```python
from build123d import *

# Parameters (mm, degrees)
BOSS_EXTRUDE1_START = -70.140187
SKETCH1_R           = 68.58
SKETCH1_R_2         = 66.04
BOSS_EXTRUDE1_DEPTH = 70.140187
SKETCH2_R           = 3.175
SKETCH2_R_2         = 63.5
BOSS_EXTRUDE2_DEPTH = 1.5875


with BuildPart() as part:
    # Sketch1 → Boss-Extrude1 (new body)
    with BuildSketch(Plane.XY.offset(BOSS_EXTRUDE1_START)):
        with Locations((24.840813797, -46.264409372)):
            Circle(SKETCH1_R)
        with Locations((24.840813797, -46.264409372)):
            Circle(SKETCH1_R_2, mode=Mode.SUBTRACT)
    extrude(amount=BOSS_EXTRUDE1_DEPTH)

    # Sketch2 → Boss-Extrude2 (add)
    with BuildSketch(Plane(origin=(0, 0, -70.14018706), x_dir=(-1, 0, 0), z_dir=(0, 0, -1))):
        Polygon((0, -107.763073453), (107.763073453, 0), (0, 107.763073453), (-107.763073453, 0), align=None)
        with Locations((0, 98.782817332)):
            Circle(SKETCH2_R, mode=Mode.SUBTRACT)
        with Locations((98.782817332, 0)):
            Circle(SKETCH2_R, mode=Mode.SUBTRACT)
        with Locations((0, -98.782817332)):
            Circle(SKETCH2_R, mode=Mode.SUBTRACT)
        with Locations((-98.782817332, 0)):
            Circle(SKETCH2_R, mode=Mode.SUBTRACT)
        with Locations(Location((0, 0, 0), (0, 0, 173.121854306))):
            Circle(SKETCH2_R_2, mode=Mode.SUBTRACT)
    extrude(amount=BOSS_EXTRUDE2_DEPTH)


solid = part.part
```
Here's how the part is built. I have some questions about the finished solid (model axes, mm). A direction names the side the tool comes from. Give positions to 0.01 mm unless a question says otherwise; leave off trailing zeros. Loops run counter-clockwise (first coordinate to the right, second up) from the corner with the lowest first, then second, coordinate; pieces in that order, holes last. Notation, with made-up numbers: M 32,32.5 L 90,32.5 A8 ccw 90,38.5 Z; hole C 70.5,20.5 d11. An arc over 180 degrees is marked long. Use one line per item in the form item = value. Start each with the question number.
Q1. I need wall thicknesses on line 1 along Y through (x, z) = (0, -71.25); line 2 along Z through (x, y) = (71.5, -27); line 3 along X through (y, z) = (-76.5, -19.5). Which ranges of each line are inside material? Lowest first, please.
Q2. Which directions (+Z, -Z, +X, -X, +Y, -Y) give clear straight access to the entire face, cutting with the end or side of a thin tool? Please do faces 1 (the flat face through (23, -62, -70.14)), 2 (the flat face through (46, -109, -70.14)), 3 (the flat face through (-10, 11, -70.14)).
Q3. If we section it at B-B (y = -37): Write out the boundary of the cut face in (x, z).
Q4. If we section it at C-C (x = 11): Write out the boundary of the cut face in (y, z).
Q5. Will these pins go through, and if not, where does the flat tip stop? pin 1 Ø5 at (x, z) = (3.5, -17) entering from -Y; pin 2 Ø7.5 at (x, y) = (0, -98.78) entering from +Z; pin 3 Ø1.5 at (x, z) = (-10, -48) entering from -Y.
Q6. If we section it at A-A (x = 81.5): Write out the boundary of the cut face in (y, z), then the cut area to 3 significant figures.
Q7. If we section it at D-D (z = -12.5): Write out the boundary of the cut face in (x, y), then the cut area to 3 significant figures.
Q8. Thinking about a two-plate mould opening in Y: for faces 4 (the cylindrical face through (-27.566, -86.449, -35.561)), 5 (the flat face through (54.636, -53.127, -70.923)), 6 (the cylindrical face through (-25.705, 0.085, -35.561)), 7 (the flat face through (-54.636, 53.127, -70.923)), which applies, +Y half, -Y half, draft (parallel to the pull), parting line (faces both ways), or undercut?
Taken from the geometry:
q1.line_1 = -107.76 to -101.96, -95.61 to -63.5, 63.5 to 95.61, 101.96 to 107.76
q1.line_2 = -71.73 to -70.14
q1.line_3 = -36.71 to -33.87, 83.55 to 86.4
q2.face_1 = +Z
q2.face_2 = -Z, -Y
q2.face_3 = -Z
q3.outline = M -70.76,-71.73 L -51.61,-71.73 L -51.61,-70.14 L -70.76,-70.14 Z; M -43.11,-70.14 L -40.55,-70.14 L -40.55,0 L -43.11,0 Z; M 51.61,-71.73 L 70.76,-71.73 L 70.76,-70.14 L 51.61,-70.14 Z; M 90.23,-70.14 L 92.79,-70.14 L 92.79,0 L 90.23,0 Z
q4.outline = M -113.43,-70.14 L -110.84,-70.14 L -110.84,0 L -113.43,0 Z; M -96.76,-71.73 L -62.54,-71.73 L -62.54,-70.14 L -96.76,-70.14 Z; M 18.31,-70.14 L 20.9,-70.14 L 20.9,0 L 18.31,0 Z; M 62.54,-71.73 L 96.76,-71.73 L 96.76,-70.14 L 62.54,-70.14 Z
q5.pin_1 = -112.21
q5.pin_2 = -70.14
q5.pin_3 = -105.77
q6.outline = M -84.9,-70.14 L -80.19,-70.14 L -80.19,0 L -84.9,0 Z; M -26.26,-71.73 L 26.26,-71.73 L 26.26,-70.14 L -7.63,-70.14 L -7.63,0 L -12.34,0 L -12.34,-70.14 L -26.26,-70.14 Z
q6.area = 744 mm^2
q7.outline = C 24.84,-46.26 d137.16; hole C 24.84,-46.26 d132.08
q7.area = 1,070 mm^2
q8.face_4 = undercut
q8.face_5 = -Y half
q8.face_6 = parting line
q8.face_7 = +Y half
